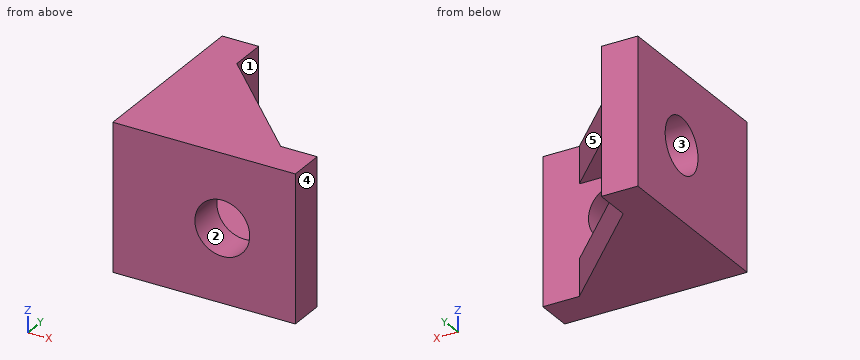
Autodesk Inventor part; units mm, degrees
ref_plane "YZ Plane" through (0, 0, 0) normal (1, 0, 0) x (0, 1, 0)
ref_plane "XZ Plane" through (0, 0, 0) normal (0, 1, 0) x (-1, 0, 0)
ref_plane "XY Plane" through (0, 0, 0) normal (0, 0, 1) x (1, 0, 0)
sketch "Boceto1" plane through (0, 0, 0) normal (0, 1, 0) x (-1, 0, 0)
  circle A0 centre (0, 0) radius 1.5
  line L0 (4, 4) -> (-4, 4)
  line L1 (-4, 4) -> (-4, -4)
  line L2 (-4, -4) -> (4, -4)
  line L3 (4, -4) -> (4, 4)
  dimension "d0" = 3
extrude "Extrusión1" add sketch "Boceto1" along normal blind 2
sketch "Boceto2" plane through (-4, 0, -4) normal (-1, 0, 0) x (0, 0, 1)
  circle A0 centre (4, 6) radius 1.5
  line L0 (8, 2) -> (8, 10)
  line L1 (8, 10) -> (0, 10)
  line L2 (0, 10) -> (0, 2)
  line L3 (8, 0) -> (0, 0)
  line L4 (0, 0) -> (8, 0)
  line L5 (8, 0) -> (8, 2)
  line L6 (0, 2) -> (0, 0)
  line L7 (0, 0) -> (8, 0)
  line L8 (8, 0) -> (8, 10)
  line L9 (8, 10) -> (0, 10)
  line L10 (0, 10) -> (0, 0)
  point P0 (4, 0)
extrude "Extrusión2" add sketch "Boceto2" along normal blind 2
sketch "Boceto3" plane through (4, 0, 4) normal (0, 0, 1) x (1, 0, 0)
  line L0 (-8, 2) -> (-8, 10)
  line L1 (-8, 10) -> (-8, 8)
  line L2 (0, 2) -> (-2, 2)
  line L3 (-2, 2) -> (-8, 8)
  line L4 (-2, 2) -> (-8, 2)
  line L5 (-8, 8) -> (-8, 2)
  point P0 (-5.5, 2)
  point P1 (-8, 4.5)
  dimension "d26" = 2
  dimension "d27" = 2
extrude "Extrusión8" add sketch "Boceto3" against normal blind 2
sketch "Boceto9" plane through (4, 0, -4) normal (0, 0, -1) x (-1, 0, 0)
  line L0 (0, 2) -> (8, 2)
  line L1 (8, 8) -> (2, 2)
  line L2 (2, 2) -> (8, 8)
  line L3 (8, 8) -> (8, 2)
  line L4 (8, 2) -> (2, 2)
  point P0 (4, 0)
extrude "Extrusión9" add sketch "Boceto9" against normal blind 2
scale "Escala1" factors (1.5, 1.5, 1.5) then translate (3, -2.5, 0) bodies 1
properties part number "Base auxiliar - esquadra"
The model under review builds one solid part; all positions refer to its coordinate system, in mm. Face numbers are marked on the shaded views. A direction names the side the tool comes from. Round coordinates to 2 decimals unless told otherwise and drop trailing zeros. Write each loop counter-clockwise with the first axis right and the second up, starting at its lowest first coordinate (ties: lowest second). Pieces come first, ordered by that corner, then holes. Notation, with made-up numbers: (19, 24.5) -> (68, 24.5) arc R28 cw to (68, 42.5) -> close; hole circle Ø11 at (-39.75, 2). An arc over 180 degrees is marked (long way). Use CSV: the item, a comma, the result in double quotes.
Q1. Consider section D-D (x = -1). Give the boundary of the cut face in (y, z), then the cut area to 3 significant figures.
Checks:
outline,"(-2.5, -6) -> (7.5, -6) -> (7.5, -3) -> (0.5, -3) -> (0.5, 3) -> (7.5, 3) -> (7.5, 6) -> (-2.5, 6) -> close"
area,"78.0 mm²"
Q2. For pin 1 Ø1.5 at (x, z) = (0, -0.5) entering from +Y; pin 2 Ø5 at (y, z) = (6.5, 0) entering from +X, all flat-tipped, find the tip position at first contact; note any pin that passes through.
Checks:
pin 1,"y = 0.5"
pin 2,"x = -3"
Q3. Mouldability with a two-part tool opening along Y and no side actions: class the marked faces 3, 4 and 5 as released by +Y, released by -Y, zero draft, split by the parting line, or undercut.
Checks:
face 3,"undercut"
face 4,"zero draft"
face 5,"released by +Y"
Q4. Consider section B-B (x = 3). Give the boundary of the cut face in (y, z).
Checks:
outline,"(-2.5, -6) -> (3.5, -6) -> (3.5, -3) -> (0.5, -3) -> (0.5, -2.25) -> (-2.5, -2.25) -> close; (-2.5, 2.25) -> (0.5, 2.25) -> (0.5, 3) -> (3.5, 3) -> (3.5, 6) -> (-2.5, 6) -> close"
Q5. Consider section C-C (z = -1.5). Give the boundary of the cut face in (x, y).
Checks:
outline,"(-6, -2.5) -> (1.32, -2.5) -> (1.32, 0.5) -> (-3, 0.5) -> (-3, 4.82) -> (-6, 4.82) -> close; (-6, 8.18) -> (-3, 8.18) -> (-3, 12.5) -> (-6, 12.5) -> close; (4.68, -2.5) -> (9, -2.5) -> (9, 0.5) -> (4.68, 0.5) -> close"
Q6. To check wall thickness, follow probe 1 along Z at (x, y) = (1, 1.5); probe 2 along Z at (x, y) = (3, -1.5); probe 3 along Y at (x, z) = (-4.8, 0). State the ranges of each line that lie inside material, in increasing order. Write a range as [from, to].
Checks:
probe 1,"[-6, -3], [3, 6]"
probe 2,"[-6, -2.25], [2.25, 6]"
probe 3,"[-2.5, 4.25], [8.75, 12.5]"
Q7. For the marked faces 1 and 2, list the 3-axis set-ups (+Z, -Z, +X, -X, +Y, -Y) from which the entire face can be reached by the end or side of a thin tool; tool diameter is ignored.
Checks:
face 1,"+X, +Y"
face 2,"+Y, -Y"
Q8. Consider section A-A (y = 6.5). Give the boundary of the cut face in (x, z), then the cut area to 3 significant figures.
Checks:
outline,"(-6, -6) -> (0, -6) -> (0, -3) -> (-3, -3) -> (-3, -2.25) -> (-6, -2.25) -> close; (-6, 2.25) -> (-3, 2.25) -> (-3, 3) -> (0, 3) -> (0, 6) -> (-6, 6) -> close"
area,"40.5 mm²"
